For this review, take the finished solid that the model builds, in its own axes (mm). Coordinates: 2 decimals unless noted, no trailing zeros. Write each loop counter-clockwise with the first axis right and the second up, starting at its lowest first coordinate (ties: lowest second). Pieces come first, ordered by that corner, then holes.
1) We need section B-B on y = 117.5. Write out the cut boundary in (x, z), then the cut area to 3 significant figures.
2) To check wall thickness, follow line 1 along Y through (x, z) = (0, -5.5); line 2 along Z through (x, y) = (0, 194.5); line 3 along Z through (x, y) = (0.75, 235.5). State the ranges of each line that lie inside material, in increasing order.
3) Insertion check: P1, Ø2, axis at y = 6.35, z = 0, coming from the +X side; P2, Ø4, axis at y = 240.5, z = 3, coming from the -X side; P3, Ø1, axis at x = -2, y = 228.5, coming from the -Z side; P4, Ø1, axis at x = -4.5, y = 61, coming from the -Z side. Each pin has a flat end and moves straight along its axis. Give the tip position at first contact, or say it passes through.
4) We need section A-A on x = 2.5. Write out the cut boundary in (y, z).
from build123d import *

# Parameters (mm, degrees)
SKETCH1_R           = 5.9944
SKETCH1_R_2         = 4.953
BOSS_EXTRUDE1_DEPTH = 304.8
CUT_EXTRUDE1_START  = -1.090901
SKETCH2_R           = 0.6985
CUT_EXTRUDE1_DEPTH  = 1.090901
CIRPATTERN1_COUNT   = 4


with BuildPart() as part:
    # Sketch1 → Boss-Extrude1 (new body)
    with BuildSketch(Plane(origin=(0, 0, 0), x_dir=(1, 0, 0), z_dir=(0, 1, 0))):
        Circle(SKETCH1_R)
        Circle(SKETCH1_R_2, mode=Mode.SUBTRACT)
    extrude(amount=BOSS_EXTRUDE1_DEPTH)

    # Sketch2 → Cut-Extrude1 (cut)
    with BuildSketch(Plane.XY.offset(5.9944).offset(CUT_EXTRUDE1_START)):
        with Locations((0, 6.35)):
            Circle(SKETCH2_R)
        with Locations((0, 19.05)):
            Circle(SKETCH2_R)
        with Locations((0, 298.45)):
            Circle(SKETCH2_R)
        with Locations((0, 285.75)):
            Circle(SKETCH2_R)
    cut_extrude1 = extrude(amount=CUT_EXTRUDE1_DEPTH, mode=Mode.SUBTRACT)

    # CirPattern1: Cut-Extrude1 ×4 about axis
    cirpattern1_axis = Axis((0, 304.8, 0), (0, 1, 0))
    for i in range(1, CIRPATTERN1_COUNT):
        add(cut_extrude1.rotate(cirpattern1_axis, i * 360 / CIRPATTERN1_COUNT), mode=Mode.SUBTRACT)


solid = part.part
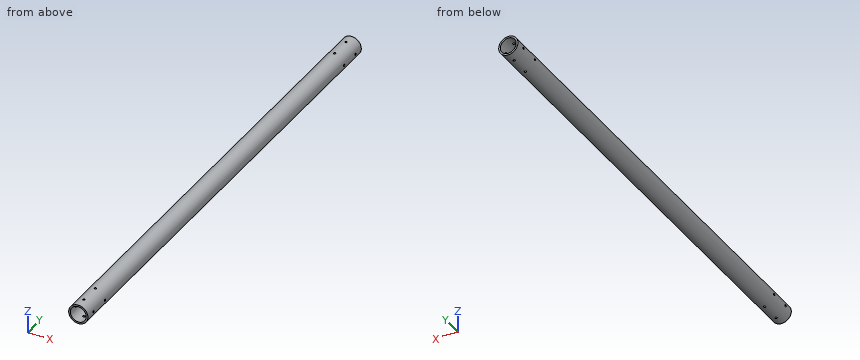
Result:
1. outline: circle Ø11.99 at (0, 0); hole circle Ø9.91 at (0, 0)
1. area: 35.8 mm2
2. line 1: y = 0 to 5.65, 7.05 to 18.35, 19.75 to 285.05, 286.45 to 297.75, 299.15 to 304.8
2. line 2: z = -5.99 to -4.95, 4.95 to 5.99
2. line 3: z = -5.95 to -4.9, 4.9 to 5.95
3. P1: stops at x = 5.99
3. P2: stops at x = -5.91
3. P3: stops at z = -5.8
3. P4: stops at z = -4.46
4. outline: (0, -5.45) - (304.8, -5.45) - (304.8, -4.28) - (0, -4.28) - close; (0, 4.28) - (304.8, 4.28) - (304.8, 5.45) - (0, 5.45) - close
